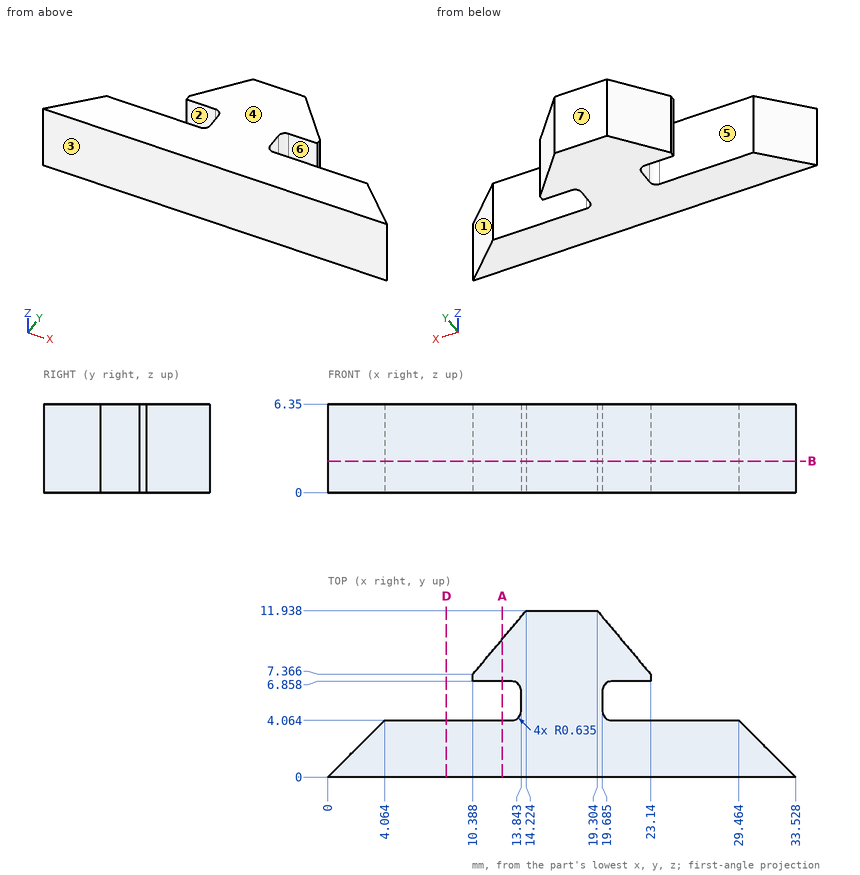
Geometry check sheet. Reference: drawing and pictorial views, mm from the part's lowest x, y, z. A direction names the side the tool comes from. Coordinates: 2 decimals unless noted, no trailing zeros. Write each loop counter-clockwise with the first axis right and the second up, starting at its lowest first coordinate (ties: lowest second). Pieces come first, ordered by that corner, then holes. Notation, with made-up numbers: (74, 66) - (93, 66) arc R36 ccw to (93, 104) - close; hole circle Ø10 at (19, -18.75). An arc over 180 degrees is marked (long way). Write item = value, one per line.
Q1. Material ranges on L1, parallel to X at y = 5, z = 4 (1 decimal); L2, parallel to Y at x = 7, z = 2.5; L3, parallel to Y at x = 13, z = 5 (1 decimal), recorded low to high. Write a range as from..to.
Answer:
L1 = 13.8..19.7
L2 = 0..4.06
L3 = 0..4.1, 6.9..10.5
Q2. Go/stop test with flat-tipped pins: pin 1 Ø1.5 at (y, z) = (3, 1.5) entering from -X; pin 2 Ø0.5 at (y, z) = (5.5, 4.5) entering from -X; pin 3 Ø1.9 at (x, z) = (22.5, 3) entering from +Y. Record where each tip stops, or that it passes through.
Answer:
pin_1 = 2.25
pin_2 = 13.84
pin_3 = 9.26
Q3. Access from +Z, -Z, +X, -X, +Y, -Y to the whole of each face (thin tool, end or side, straight path). Record for the marked faces 5, 6 and 7.
Answer:
face_5 = +Z, -Z, -X
face_6 = +Z, -Z, +X
face_7 = +Z, -Z, +X, -X, +Y
Q4. Cross-section at D-D (x = 8.5). Enter the section's corners in (y, z).
Answer:
outline = (0, 0) - (4.06, 0) - (4.06, 6.35) - (0, 6.35) - close
Q5. Mould release check, pull along Y, two halves, no side actions. Record for the marked faces 1, 2, 3 and 4: released by +Y, released by -Y, zero draft, split by the parting line, or undercut.
Answer:
face_1 = released by +Y
face_2 = undercut
face_3 = released by -Y
face_4 = zero draft
Q6. Cross-section at B-B (z = 2.25). Enter the section's corners in (x, y) (1 decimal), plus the area to 3 significant figures.
Answer:
outline = (0, 0) - (33.5, 0) - (29.5, 4.1) - (20.3, 4.1) arc R0.6 cw to (19.7, 4.7) - (19.7, 6.2) arc R0.6 cw to (20.3, 6.9) - (23.1, 6.9) - (23.1, 7.4) - (19.3, 11.9) - (14.2, 11.9) - (10.4, 7.4) - (10.4, 6.9) - (13.2, 6.9) arc R0.6 cw to (13.8, 6.2) - (13.8, 4.7) arc R0.6 cw to (13.2, 4.1) - (4.1, 4.1) - close
area = 184 mm²
Q7. Cross-section at A-A (x = 12.5). Enter the section's corners in (y, z).
Answer:
outline = (0, 0) - (4.06, 0) - (4.06, 6.35) - (0, 6.35) - close; (6.86, 0) - (9.88, 0) - (9.88, 6.35) - (6.86, 6.35) - close
